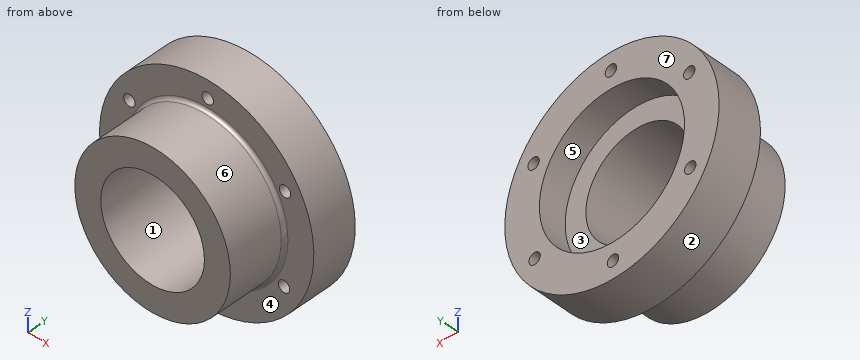
from build123d import *

# Parameters (mm, degrees)
ESBO_O1_R                = 31
RESSALTO_EXTRUS_O1_DEPTH = 30
ESBO_O2_R                = 31
ESBO_O2_R_2              = 22.5
CORTE_EXTRUS_O1_DEPTH    = 17
ESBO_O2_3_R              = 15
CORTE_EXTRUS_O2_DEPTH    = 54.122499941
ESBO_O4_R                = 21
CORTE_EXTRUS_O3_DEPTH    = 8.1
FURO_ROSCADO_DE_M41_D    = 3.3
FILETE1_R                = 1


with BuildPart() as part:
    # Esbo_o1 → Ressalto-extrus_o1 (new body)
    with BuildSketch(Plane(origin=(0, 0, 0), x_dir=(1, 0, 0), z_dir=(0, 1, 0))):
        with Locations(Location((0, 0, 0), (0, 0, 270))):
            Circle(ESBO_O1_R)
    extrude(amount=RESSALTO_EXTRUS_O1_DEPTH)

    # Esbo_o2 → Corte-extrus_o1 (cut)
    with BuildSketch(Plane.XZ):
        with Locations(Location((0, 0, 0), (0, 0, 270))):
            Circle(ESBO_O2_R)
        with Locations(Location((0, 0, 0), (0, 0, 270))):
            Circle(ESBO_O2_R_2, mode=Mode.SUBTRACT)
    extrude(amount=-CORTE_EXTRUS_O1_DEPTH, mode=Mode.SUBTRACT)

    # Esbo_o2_3 → Corte-extrus_o2 (cut, through all)
    with BuildSketch(Plane.XZ):
        with Locations(Location((0, 0, 0), (0, 0, 270))):
            Circle(ESBO_O2_3_R)
    extrude(amount=-CORTE_EXTRUS_O2_DEPTH, mode=Mode.SUBTRACT)

    # Esbo_o4 → Corte-extrus_o3 (cut)
    with BuildSketch(Plane(origin=(0, 30, 0), x_dir=(1, 0, 0), z_dir=(0, 1, 0))):
        with Locations(Location((0, 0, 0), (0, 0, 270))):
            Circle(ESBO_O4_R)
    extrude(amount=-CORTE_EXTRUS_O3_DEPTH, mode=Mode.SUBTRACT)

    # Furo roscado de M41 (through all)
    with Locations(Plane(origin=(0, 30, 0), x_dir=(1, 0, 0), z_dir=(0, 1, 0))):
        with Locations((-0.294790254, 25.998328768), (22.367818042, 13.254460232), (22.662608295, -12.743868535), (0.294790254, -25.998328768), (-22.367818042, -13.254460232), (-22.662608295, 12.743868535)):
            Hole(FURO_ROSCADO_DE_M41_D / 2)

    # Filete1
    filete1_edges = [part.edges().sort_by_distance(p)[0] for p in [
        (0, 17, 22.5),
    ]]
    fillet(filete1_edges, radius=FILETE1_R)


solid = part.part
The listing builds one solid part. Answer for the finished solid, in the listing's coordinates (mm). Face numbers are marked on the shaded views. A direction names the side the tool comes from. Coordinates: 2 decimals unless noted, no trailing zeros. Order: outer loops, then holes, each group sorted by start corner. A loop starts at its lowest first (then second) coordinate and runs counter-clockwise, first axis right, second up.
Q1. Given P1, Ø5.5, axis at x = 0.29, z = 26, coming from the -Y side; P2, Ø5, axis at x = 12, y = 13, coming from the -Z side; P3, Ø4, axis at y = 24.5, z = -20.5, coming from the +X side; P4, Ø5, axis at x = -5.5, z = -20.5, coming from the -Y side, each flat-ended and moving along its own axis, determine where each tip first touches the part or whether it passes through.
Q2. Which of the six approach directions +Z, -Z, +X, -X, +Y, -Y give full straight-line access (tool end or side, diameter ignored) to the marked faces 5, 6 and 7?
Q3. A cutting plane is placed at B-B, the plane x = 0. Write down the section's boundary in (y, z), and give its area (3 significant figures).
Q4. A cutting plane is placed at A-A, the plane z = 0. Write down the section's boundary in (x, y), and give its area (3 significant figures).
Q5. Consider line 1 (X direction, y = 22, z = 13); line 2 (X direction, y = 25.25, z = 0); line 3 (X direction, y = 7.75, z = 0). Determine where each line is inside the solid, lowest interval first.
Q6. A cutting plane is placed at D-D, the plane y = 20.75. Write down the section's boundary in (x, z).
Q7. For a pull along Z with two mould halves and no side action, classify the marked faces 1, 2, 3 and 4 as pulls with the +Z half, pulls with the -Z half, needs draft (parallel to the pull), parting line crosses it, or undercut.
Q8. A cutting plane is placed at C-C, the plane y = 15.25. Write down the section's boundary in (x, z), and give its area (3 significant figures).
Answers follow:
1. P1: stops at y = 16.97
1. P2: stops at z = -20.4
1. P3: stops at x = 24.87
1. P4: stops at y = 0
2. face 5: +Y
2. face 6: -Y
2. face 7: +Z, -Z, +X, -X, +Y
3. outline: (0, -22.5) - (16, -22.5) arc R1 cw to (17, -23.5) - (17, -24.37) - (30, -24.37) - (30, -21) - (21.9, -21) - (21.9, -15) - (0, -15) - close; (0, 15) - (21.9, 15) - (21.9, 21) - (30, 21) - (30, 24.37) - (17, 24.37) - (17, 23.5) arc R1 cw to (16, 22.5) - (0, 22.5) - close; (17, -31) - (30, -31) - (30, -27.62) - (17, -27.62) - close; (17, 27.62) - (30, 27.62) - (30, 31) - (17, 31) - close
3. area: 490 mm2
4. outline: (-31, 17) - (-23.5, 17) arc R1 cw to (-22.5, 16) - (-22.5, 0) - (-15, 0) - (-15, 21.9) - (-21, 21.9) - (-21, 30) - (-31, 30) - close; (15, 0) - (22.5, 0) - (22.5, 16) arc R1 cw to (23.5, 17) - (31, 17) - (31, 30) - (21, 30) - (21, 21.9) - (15, 21.9) - close
4. area: 574 mm2
5. line 1: x = -28.14 to -24, -20.74 to -16.49, 16.49 to 21.03, 24.29 to 28.14
5. line 2: x = -31 to -21, 21 to 31
5. line 3: x = -22.5 to -15, 15 to 22.5
6. outline: circle Ø62 at (0, 0); hole circle Ø3.3 at (-22.66, -12.74); hole circle Ø3.3 at (-22.37, 13.25); hole circle Ø30 at (0, 0); hole circle Ø3.3 at (-0.29, -26); hole circle Ø3.3 at (0.29, 26); hole circle Ø3.3 at (22.37, -13.25); hole circle Ø3.3 at (22.66, 12.74)
7. face 1: undercut
7. face 2: parting line crosses it
7. face 3: undercut
7. face 4: needs draft
8. outline: circle Ø45 at (0, 0); hole circle Ø30 at (0, 0)
8. area: 884 mm2
